Can you work these out from the model? Positions are in its coordinate system, mm. Face numbers are marked on the shaded views. A direction names the side the tool comes from. Give positions to 0.01 mm unless a question says otherwise; leave off trailing zeros. Loops run counter-clockwise (first coordinate to the right, second up) from the corner with the lowest first, then second, coordinate; pieces in that order, holes last. Notation, with made-up numbers: (33, 17) - (75, 17) arc R24 ccw to (75, 34) - close; hole circle Ø11 at (82, 24). An arc over 180 degrees is marked (long way). Answer as a JSON object with one key per item and string values. Group by question number.
Item 1: Suppose I cut it at D-D on x = 0. Write out the boundary of the cut face in (y, z), and give its area (3 significant figures).
Item 2: Please list where these lines run through material, in increasing order: L1, parallel to X at y = -10.5, z = 4.5; L2, parallel to Y at x = -60, z = 22; L3, parallel to Z at x = -62.5, y = -16.5.
Item 3: Which directions (+Z, -Z, +X, -X, +Y, -Y) give clear straight access to the entire face, cutting with the end or side of a thin tool? Please do the marked faces 1, 2, 3 and 4.
Item 4: Suppose I cut it at B-B on x = -31.75. Write out the boundary of the cut face in (y, z), and give its area (3 significant figures).
Item 5: Suppose I cut it at A-A on z = 22. Write out the boundary of the cut face in (x, y).
Item 6: Will these pins go through, and if not, where does the flat tip stop? pin 1 (1 mm diameter, centred on x = 53.5, y = -5.5, fed in from +Z); pin 2 (7 mm diameter, centred on x = 60, y = -12.5, fed in from -Z); pin 3 (7.5 mm diameter, centred on x = 31.75, z = -27.25, fed in from -Y); pin 4 (11 mm diameter, centred on x = 60, y = -12.5, fed in from -Z).
Item 7: Thinking about a two-plate mould opening in Z: for the marked faces 5, 6 and 7, which applies, pulls with the +Z half, pulls with the -Z half, needs draft (parallel to the pull), parting line crosses it, or undercut?
Item 8: Suppose I cut it at C-C on y = -12.5. Count the separate pieces of the cut face and the enclosed holes in it, and give its area (3 significant figures).
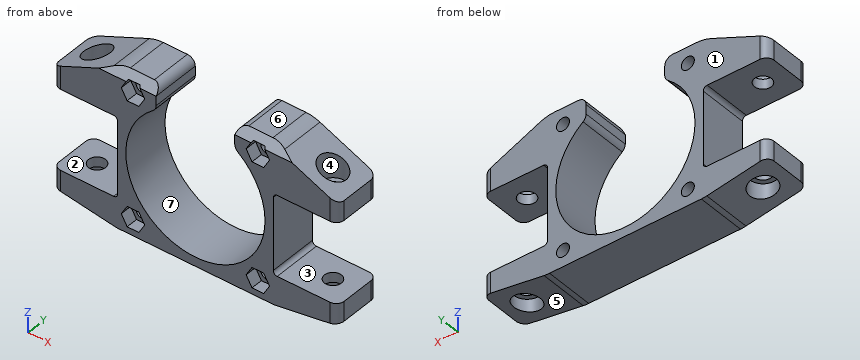
from build123d import *

# Parameters (mm, degrees)
PAD_DEPTH         = 25
SKETCH001_R       = 4.3
POCKET_DEPTH      = 100
POCKET_DEPTH_BACK = -100
SKETCH002_R       = 6.75
POCKET001_DEPTH   = 10.101
SKETCH003_R       = 6.75
POCKET002_DEPTH   = 19.101
SKETCH004_R       = 3.3
POCKET003_DEPTH   = 25.001
POCKET004_DEPTH   = 6
FILLET_R          = 4
FILLET001_R       = 2
FILLET002_R       = 18
FILLET003_R       = 4
POCKET005_DEPTH   = 145.001


with BuildPart() as part:
    # Sketch → Pad (new body)
    with BuildSketch(Plane.XZ):
        with BuildLine():
            Line((-72.5, 20.4), (-72.5, 30.4))
            Line((-72.5, 30.4), (-40, 44.5))
            Line((-40, 44.5), (-20, 44.5))
            Line((-20, 44.5), (-20, 33.708903))
            ThreePointArc((-20, 33.708903), (0, -30.9), (20, 33.708903))
            Line((20, 44.5), (20, 33.708903))
            Line((40, 44.5), (20, 44.5))
            Line((40, 44.5), (72.5, 30.4))
            Line((72.5, 30.4), (72.5, 20.4))
            Line((72.5, 20.4), (39.6, 20.4))
            Line((39.6, 20.4), (39.6, -20.4))
            Line((39.6, -20.4), (72.5, -20.4))
            Line((72.5, -20.4), (72.5, -30.4))
            Line((72.5, -30.4), (40, -35.5))
            Line((40, -35.5), (-40, -35.5))
            Line((-40, -35.5), (-72.5, -30.4))
            Line((-72.5, -30.4), (-72.5, -20.4))
            Line((-72.5, -20.4), (-39.6, -20.4))
            Line((-39.6, -20.4), (-39.6, 20.4))
            Line((-39.6, 20.4), (-72.5, 20.4))
        make_face()
    extrude(amount=PAD_DEPTH)

    # Sketch001 (on Face11 of Pad) → Pocket (cut, two sides)
    with BuildSketch(Plane(origin=(0, 0, -20.4), x_dir=(-1, 0, 0), z_dir=(0, 0, 1))) as pocket_sk:
        with Locations((-60, 12.5)):
            Circle(SKETCH001_R)
        with Locations((60, 12.5)):
            Circle(SKETCH001_R)
    extrude(amount=-POCKET_DEPTH, mode=Mode.SUBTRACT)
    extrude(pocket_sk.sketch, amount=-POCKET_DEPTH_BACK, mode=Mode.SUBTRACT)

    # Sketch002 (on Face16 of Pocket) → Pocket001 (cut, through all)
    with BuildSketch(Plane(origin=(0, 0, -25.4), x_dir=(-1, 0, 0), z_dir=(0, 0, 1))):
        with Locations((-60, 12.5)):
            Circle(SKETCH002_R)
        with Locations((60, 12.5)):
            Circle(SKETCH002_R)
    extrude(amount=-POCKET001_DEPTH, mode=Mode.SUBTRACT)

    # Sketch003 (on Face16 of Pocket001) → Pocket002 (cut, through all)
    with BuildSketch(Plane(origin=(0, 0, 25.4), x_dir=(-1, 0, 0), z_dir=(0, 0, 1))):
        with Locations((-60, 12.5)):
            Circle(SKETCH003_R)
        with Locations((60, 12.5)):
            Circle(SKETCH003_R)
    extrude(amount=POCKET002_DEPTH, mode=Mode.SUBTRACT)

    # Sketch004 (on Face4 of Pocket002) → Pocket003 (cut, through all)
    with BuildSketch(Plane.XZ.offset(25)):
        with Locations((-31.75, 36.25)):
            Circle(SKETCH004_R)
        with Locations((31.75, 36.25)):
            Circle(SKETCH004_R)
        with Locations((31.75, -27.25)):
            Circle(SKETCH004_R)
        with Locations((-31.75, -27.25)):
            Circle(SKETCH004_R)
    extrude(amount=-POCKET003_DEPTH, mode=Mode.SUBTRACT)

    # Sketch005 (on Face4 of Pocket003) → Pocket004 (cut)
    with BuildSketch(Plane.XZ.offset(25)):
        Polygon((-25.803292, 36.25), (-28.776646, 41.4), (-34.723354, 41.4), (-37.696708, 36.25), (-34.723354, 31.1), (-28.776646, 31.1), align=None)
        Polygon((34.723354, 31.1), (37.696708, 36.25), (34.723354, 41.4), (28.776646, 41.4), (25.803292, 36.25), (28.776646, 31.1), align=None)
        Polygon((28.776646, -32.4), (34.723354, -32.4), (37.696708, -27.25), (34.723354, -22.1), (28.776646, -22.1), (25.803292, -27.25), align=None)
        Polygon((-28.776646, -32.4), (-25.803292, -27.25), (-28.776646, -22.1), (-34.723354, -22.1), (-37.696708, -27.25), (-34.723354, -32.4), align=None)
    extrude(amount=-POCKET004_DEPTH, mode=Mode.SUBTRACT)

    # Fillet
    fillet_edges = [part.edges().sort_by_distance(p)[0] for p in [
        (72.5, -25, 25.4),
        (72.5, 0, 25.4),
        (72.5, -25, -25.4),
        (72.5, 0, -25.4),
        (-72.5, -25, 25.4),
        (-72.5, -25, -25.4),
        (-72.5, 0, 25.4),
        (-72.5, 0, -25.4),
    ]]
    fillet(fillet_edges, radius=FILLET_R)

    # Fillet001
    fillet001_edges = [part.edges().sort_by_distance(p)[0] for p in [
        (-39.6, -12.5, -20.4),
        (-39.6, -12.5, 20.4),
        (39.6, -12.5, -20.4),
        (39.6, -12.5, 20.4),
    ]]
    fillet(fillet001_edges, radius=FILLET001_R)

    # Fillet002
    fillet002_edges = [part.edges().sort_by_distance(p)[0] for p in [
        (40, -12.5, 44.5),
        (-40, -12.5, 44.5),
        (40, -12.5, -35.5),
        (-40, -12.5, -35.5),
    ]]
    fillet(fillet002_edges, radius=FILLET002_R)

    # Fillet003
    fillet003_edges = [part.edges().sort_by_distance(p)[0] for p in [
        (-20, -12.5, 44.5),
        (-20, -12.5, 33.708903),
        (20, -12.5, 44.5),
        (20, -12.5, 33.708903),
    ]]
    fillet(fillet003_edges, radius=FILLET003_R)

    # Sketch006 (on Face39 of Fillet003) → Pocket005 (cut, through all)
    with BuildSketch(Plane(origin=(72.5, 0, 0), x_dir=(0, 0, 1), z_dir=(1, 0, 0))):
        Polygon((40.5, 25), (44.5, 21), (44.5, 25), align=None)
    extrude(amount=-POCKET005_DEPTH, mode=Mode.SUBTRACT)


solid = part.part
Worked out:
{
 "1": {"outline": "(-25, -35.5) - (0, -35.5) - (0, -30.9) - (-25, -30.9) - close", "area": "115 mm2"},
 "2": {"L1": "x = -39.6 to -35.4, 35.4 to 39.6", "L2": "y = -25 to -16.8, -8.2 to 0", "L3": "z = -25.4 to -20.4, 20.4 to 25.4"},
 "3": {"face 1": "+Z, -Z, +X, -X, +Y", "face 2": "-X, +Y, -Y", "face 3": "+X, +Y, -Y", "face 4": "+Z"},
 "4": {"outline": "(-25, -35.5) - (0, -35.5) - (0, -30.55) - (-19, -30.55) - (-19, -32.4) - (-25, -32.4) - close; (-25, -22.1) - (-19, -22.1) - (-19, -23.95) - (0, -23.95) - (0, -11.16) - (-25, -11.16) - close; (-25, 20.16) - (0, 20.16) - (0, 32.95) - (-19, 32.95) - (-19, 31.1) - (-25, 31.1) - close; (-24.1, 41.4) - (-19, 41.4) - (-19, 39.55) - (0, 39.55) - (0, 44.5) - (-21, 44.5) - close", "area": "835 mm2"},
 "5": {"outline": "(-72.5, -21) arc R4 ccw to (-68.5, -25) - (-30.77, -25) - (-30.77, 0) - (-68.5, 0) arc R4 ccw to (-72.5, -4) - close; (30.77, -25) - (68.5, -25) arc R4 ccw to (72.5, -21) - (72.5, -4) arc R4 ccw to (68.5, 0) - (30.77, 0) - close; hole circle Ø8.6 at (-60, -12.5); hole circle Ø8.6 at (60, -12.5)"},
 "6": {"pin 1": "stops at z = 38.86", "pin 2": "passes through", "pin 3": "stops at y = -19", "pin 4": "stops at z = -25.4"},
 "7": {"face 5": "pulls with the -Z half", "face 6": "pulls with the +Z half", "face 7": "undercut"},
 "8": {"separate pieces": "5", "enclosed holes": "4", "area": "3,310 mm2"}
}
